Autodesk Inventor part; units mm, degrees
ref_plane "YZ Plane" through (0, 0, 0) normal (1, 0, 0) x (0, 1, 0)
ref_plane "XZ Plane" through (0, 0, 0) normal (0, 1, 0) x (-1, 0, 0)
ref_plane "XY Plane" through (0, 0, 0) normal (0, 0, 1) x (1, 0, 0)
sketch "Sketch1" plane through (0, 0, 0) normal (0, 0, 1) x (1, 0, 0)
  line L0 (50.8, 0) -> (50.8, 39.0312) construction
  line L1 (0, 0) -> (49.8475, 0)
  line L2 (44.45, 0) -> (44.45, 51.6727)
  line L3 (0, 0) -> (0, 50.5742)
  line L4 (49.8475, 0) -> (49.8475, 45.6895)
  line L5 (49.8475, 4.7625) -> (44.45, 4.7625)
  line L6 (44.45, 11.1125) -> (49.8475, 11.1125)
  line L7 (49.8475, 30.1625) -> (44.45, 30.1625)
  line L8 (44.45, 36.5125) -> (49.8475, 36.5125)
  line L9 (49.8475, 41.275) -> (0, 41.275)
  line L10 (11.8237, 0) -> (11.8237, 53.9909)
  line L11 (15.875, 0) -> (15.875, 48.05)
  line L12 (11.8237, 4.7625) -> (15.875, 4.7625)
  line L13 (15.875, 9.5377) -> (11.8237, 9.5377)
  line L14 (15.875, 31.7373) -> (11.8237, 31.7373)
  line L15 (11.8237, 36.5125) -> (15.875, 36.5125)
  point P0 (47.1487, 36.5125)
  point P1 (44.45, 30.1625)
  point P2 (11.8237, 41.275)
  dimension "d1" = 49.8475
  dimension "d2" = 44.45
  dimension "d3" = 6.35
  dimension "d4" = 6.35
  dimension "d5" = 4.7625
  dimension "d6" = 19.05
  dimension "d7" = 4.7625
  dimension "d12" = 41.275
  dimension "d20" = 11.8237
  dimension "d21" = 5.3975
  dimension "d22" = 15.875
  dimension "d23" = 4.7752
  dimension "d24" = 4.7752
revolve "Revolution1" add sketch "Sketch1" angle 360 about axis through (0, 0, 0) along (0, 1, 0) contours L10 L12 L11 L1 | L11 L9 L2 L1 | L9 L11 L15 L10 | L2 L5 L4 L1 | L10 L14 L11 L13 | L9 L4 L8 L2 | L2 L7 L4 L6
chamfer "Chamfer1" distance 0.635 angle 45 12 edges at (-49.8475, 0, 0) (-49.8475, 4.7625, 0) (-49.8475, 11.1125, 0) (-49.8475, 30.1625, 0) (-49.8475, 36.5125, 0) (-49.8475, 41.275, 0) (-11.8237, 41.275, 0) (-11.8237, 36.5125, 0) (-11.8237, 31.7373, 0) (-11.8237, 9.5377, 0) (-11.8237, 4.7625, 0) (-11.8237, 0, 0)
sketch "Sketch3" plane through (0, 41.275, 0) normal (0, 1, 0) x (1, 0, 0)
  circle A0 centre (0, 31.75) radius 5.3578
  circle A1 centre (-31.75, 0) radius 5.3578
  circle A2 centre (0, -31.75) radius 5.3578
  circle A3 centre (31.75, 0) radius 5.3578
  circle A4 centre (0, 0) radius 31.75 construction
  line L0 (0, 0) -> (22.4506, 22.4506) construction
  line L1 (0, 0) -> (31.75, 0) construction
  circle A5 centre (22.4506, 22.4506) radius 5.5563
  dimension "d27" = 360
  dimension "d29" = 10.7156
  dimension "d30" = 31.75
  dimension "d31" = 45
  dimension "d32" = 11.1125
extrude "Extrusion3" cut sketch "Sketch3" against normal up to surface (30.1625 mm away) contours A0 | A1 | A2 | A3
extrude "Extrusion4" cut sketch "Sketch3" against normal blind 352.425 contours A5
chamfer "Chamfer2" distance 0.635 angle 45 5 edges at (-37.1078, 41.275, 0) (-5.3578, 41.275, -31.75) (16.8944, 41.275, -22.4506) (26.3922, 41.275, 0) (-5.3578, 41.275, 31.75)
properties part number "2 Piston"
The listing builds one solid part. Answer for the finished solid, in the listing's coordinates (mm). A direction names the side the tool comes from. Round coordinates to 2 decimals unless told otherwise and drop trailing zeros. Return JSON: item names as keys, results as strings. Group by question number.
1. The mould has two halves that part along Z. Classify faces 4 (the cylindrical face through (-3.441, 34.158, 15.497)), 5 (the flat face through (-37, 4.762, 25)), 6 (the cylindrical face through (42.397, 7.982, -13.352)): pulls with the +Z half, pulls with the -Z half, needs draft (parallel to the pull), parting line crosses it, or undercut.
2. Which of the six approach directions +Z, -Z, +X, -X, +Y, -Y give full straight-line access (tool end or side, diameter ignored) to faces 1 (the flat face through (0, 11.112, -32)), 2 (the cylindrical face through (-2.563, 2.406, 11.543)), 3 (the flat face through (7, 9.538, 11))?
3. The part is cut by section A-A on y = 16.5. State how many separate pieces and enclosed holes the cut face has, then the cut area to 3 significant figures.
4. Consider probe 1 along X at (y, z) = (39, 0); probe 2 along X at (y, z) = (34.95, 0) (3 decimals). Determine where each line is inside the solid, lowest interval first.
5. Each of these flat-tipped pins is pushed along its axis until it touches: P1, Ø5, axis at x = -4.5, y = 19.5, coming from the +Z side; P2, Ø12.5, axis at x = 31.75, z = 0, coming from the +Y side (3 decimals); P3, Ø10, axis at x = 22.45, z = -22.45, coming from the -Y side; P4, Ø4, axis at y = 13.5, z = -4.5, coming from the +X side. Where does it stop, or does it pass through?
Resolved:
{
 "1": {"face 4": "undercut", "face 5": "needs draft", "face 6": "parting line crosses it"},
 "2": {"face 1": "+Y", "face 2": "+Y, -Y", "face 3": "none"},
 "3": {"separate pieces": "1", "enclosed holes": "6", "area": "6,910 mm²"},
 "4": {"probe 1": "x = -49.85 to -37.11, -26.39 to -11.82, 11.82 to 26.39, 37.11 to 49.85", "probe 2": "x = -44.45 to -37.108, -26.392 to -15.875, 15.875 to 26.392, 37.108 to 44.45"},
 "5": {"P1": "stops at z = 49.81", "P2": "stops at y = 41.275", "P3": "passes through", "P4": "stops at x = 49.78"}
}
